Check sheet for the modelled part. Datum: model origin and axes. Units: mm. Face numbers are marked on the shaded views. A direction names the side the tool comes from. Give positions to 0.01 mm unless a question says otherwise; leave off trailing zeros. Order: outer loops, then holes, each group sorted by start corner. A loop starts at its lowest first (then second) coordinate and runs counter-clockwise, first axis right, second up.
Item 1: Gauge pin test, flat ends, axial feed: P1, Ø1.9, axis at y = 8, z = 1, coming from the -X side; P2, Ø2, axis at y = 31, z = -1.5, coming from the -X side; P3, Ø1.5, axis at y = 1.5, z = 0, coming from the +X side. Record the tip position at first contact, or that the pin passes through.
Item 2: Sectioned sample at D-D on x = -4.5. Record the boundary of the cut face in (y, z) (3 decimals), and give its area (3 significant figures).
Item 3: Sectioned sample at A-A on y = 0. Record the boundary of the cut face in (x, z) (3 decimals).
Item 4: Sectioned sample at C-C on z = 0. Record the boundary of the cut face in (x, y).
Item 5: Release check for a two-part mould opening along X. For the marked faces 3, 4 and 5 record: released by +X, released by -X, zero draft, split by the parting line, or undercut.
Item 6: Sectioned sample at B-B on y = 37.5. Record the boundary of the cut face in (x, z) (3 decimals), and give its area (3 significant figures).
Item 7: Material ranges on line 1 along Y through (x, z) = (-0.1, 0); line 2 along Z through (x, y) = (3.85, 37.5) (3 decimals); line 3 along X through (y, z) = (13, 0), recorded low to high.
Item 8: Access from +Z, -Z, +X, -X, +Y, -Y to the whole of each face (thin tool, end or side, straight path). Record for the marked faces 1 and 2.
from build123d import *

# Parameters (mm, degrees)
BOSS_EXTRUDE1_DEPTH     = 3.175
CUT_EXTRUDE1_DEPTH      = 42.022196735
CUT_EXTRUDE1_DEPTH_BACK = 42.022196735
SKETCH2_R               = 1.7
SKETCH2_R_2             = 1.6


with BuildPart() as part:
    # Sketch1 → Boss-Extrude1 (new, symmetric)
    with BuildSketch(Plane.XY):
        Polygon((-2.5, -3), (2.5, -3), (2.5, 30.5), (5.7, 32.5), (5.7, 40.5), (2.7, 40.5), (2.7, 34.5), (-2.7, 34.5), (-2.7, 40.5), (-5.7, 40.5), (-5.7, 32.5), (-2.5, 30.5), align=None)
    extrude(amount=BOSS_EXTRUDE1_DEPTH, both=True)

    # Sketch2 → Cut-Extrude1 (cut, two sides: drawn at the far end of the back side and taken through both)
    with BuildSketch(Plane(origin=(0, 0, 0), x_dir=(0, 0, -1), z_dir=(1, 0, 0)).offset(-CUT_EXTRUDE1_DEPTH_BACK)):
        Circle(SKETCH2_R)
        with Locations((0, 37.5)):
            Circle(SKETCH2_R_2)
    extrude(amount=CUT_EXTRUDE1_DEPTH + CUT_EXTRUDE1_DEPTH_BACK, mode=Mode.SUBTRACT)


solid = part.part
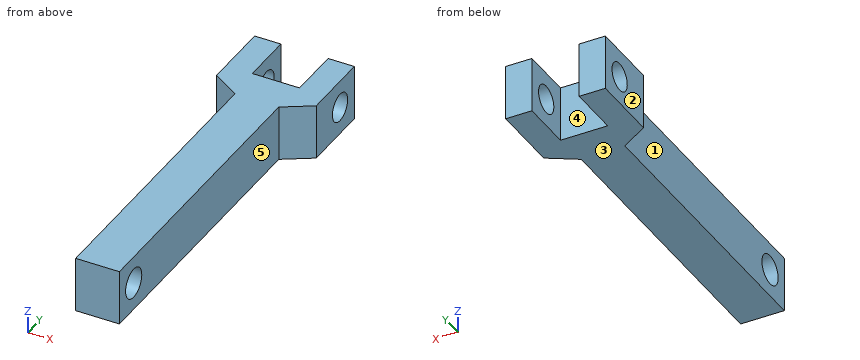
Report:
1. P1: stops at x = -2.5
1. P2: stops at x = -4.9
1. P3: stops at x = 2.5
2. outline: (31.75, -3.175) - (40.5, -3.175) - (40.5, 3.175) - (31.75, 3.175) - close; hole circle Ø3.2 at (37.5, 0)
2. area: 47.5 mm2
3. outline: (-2.5, -3.175) - (2.5, -3.175) - (2.5, -1.7) - (-2.5, -1.7) - close; (-2.5, 1.7) - (2.5, 1.7) - (2.5, 3.175) - (-2.5, 3.175) - close
4. outline: (-5.7, 32.5) - (-2.5, 30.5) - (-2.5, 1.7) - (2.5, 1.7) - (2.5, 30.5) - (5.7, 32.5) - (5.7, 35.9) - (2.7, 35.9) - (2.7, 34.5) - (-2.7, 34.5) - (-2.7, 35.9) - (-5.7, 35.9) - close; (-5.7, 39.1) - (-2.7, 39.1) - (-2.7, 40.5) - (-5.7, 40.5) - close; (-2.5, -3) - (2.5, -3) - (2.5, -1.7) - (-2.5, -1.7) - close; (2.7, 39.1) - (5.7, 39.1) - (5.7, 40.5) - (2.7, 40.5) - close
5. face 3: zero draft
5. face 4: undercut
5. face 5: released by +X
6. outline: (-5.7, -3.175) - (-2.7, -3.175) - (-2.7, -1.6) - (-5.7, -1.6) - close; (-5.7, 1.6) - (-2.7, 1.6) - (-2.7, 3.175) - (-5.7, 3.175) - close; (2.7, -3.175) - (5.7, -3.175) - (5.7, -1.6) - (2.7, -1.6) - close; (2.7, 1.6) - (5.7, 1.6) - (5.7, 3.175) - (2.7, 3.175) - close
6. area: 18.9 mm2
7. line 1: y = -3 to -1.7, 1.7 to 34.5
7. line 2: z = -3.175 to -1.6, 1.6 to 3.175
7. line 3: x = -2.5 to 2.5
8. face 1: +Z, -Z, -X, -Y
8. face 2: +Z, -Z, -X, +Y, -Y
